Part model, mm, in its own coordinate system. Face numbers are marked on the shaded views. A direction names the side the tool comes from. Coordinates: 2 decimals unless noted, no trailing zeros. Use a Markdown table: item, result.
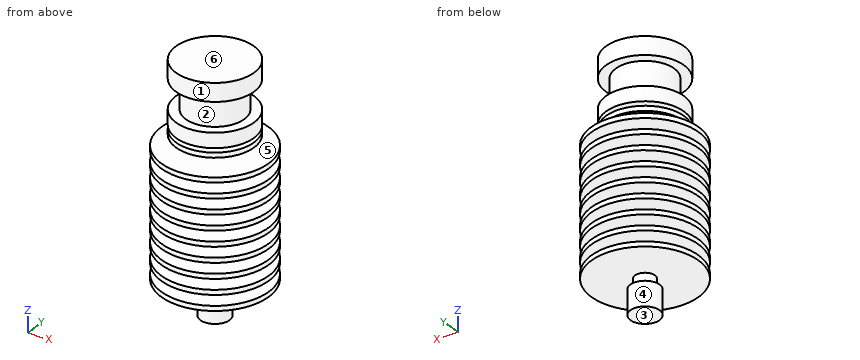
Autodesk Inventor part; units mm, degrees
ref_plane "YZ Plane" through (0, 0, 0) normal (1, 0, 0) x (0, 1, 0)
ref_plane "XZ Plane" through (0, 0, 0) normal (0, 1, 0) x (-1, 0, 0)
ref_plane "XY Plane" through (0, 0, 0) normal (0, 0, 1) x (1, 0, 0)
sketch "Sketch1" plane through (0, 0, 0) normal (1, 0, 0) x (0, 1, 0)
  line L0 (0, -49.8) -> (0, 0)
  line L1 (0, 0) -> (-8, 0)
  line L2 (-8, 0) -> (-8, -3.7)
  line L3 (-8, -3.7) -> (-6, -3.7)
  line L4 (-6, -3.7) -> (-6, -9.7)
  line L5 (-6, -9.7) -> (-8, -9.7)
  line L6 (-8, -9.7) -> (-8, -12.7)
  line L7 (-8, -12.7) -> (-3, -12.7)
  line L8 (-3, -12.7) -> (-3, -49.8)
  line L9 (-3, -49.8) -> (0, -49.8)
  line L10 (-3, -42.7) -> (-11, -42.7)
  line L11 (-11, -42.7) -> (-11, -41.7)
  line L12 (-11, -41.7) -> (-3, -41.7)
  line L13 (-3, -41.7) -> (-3, -42.7)
  line L14 (-3, -39.575) -> (-11, -39.575)
  line L15 (-11, -39.575) -> (-11, -38.575)
  line L16 (-11, -38.575) -> (-3, -38.575)
  line L17 (-3, -38.575) -> (-3, -39.575)
  line L18 (-3, -27.075) -> (-11, -27.075)
  line L19 (-11, -27.075) -> (-11, -26.075)
  line L20 (-11, -26.075) -> (-3, -26.075)
  line L21 (-3, -26.075) -> (-3, -27.075)
  line L22 (-3, -20.825) -> (-11, -20.825)
  line L23 (-11, -20.825) -> (-11, -19.825)
  line L24 (-11, -19.825) -> (-3, -19.825)
  line L25 (-3, -19.825) -> (-3, -20.825)
  line L26 (-3, -30.2) -> (-11, -30.2)
  line L27 (-11, -30.2) -> (-11, -29.2)
  line L28 (-11, -29.2) -> (-3, -29.2)
  line L29 (-3, -29.2) -> (-3, -30.2)
  line L30 (-3, -33.325) -> (-11, -33.325)
  line L31 (-11, -33.325) -> (-11, -32.325)
  line L32 (-11, -32.325) -> (-3, -32.325)
  line L33 (-3, -32.325) -> (-3, -33.325)
  line L34 (-3, -36.45) -> (-11, -36.45)
  line L35 (-11, -36.45) -> (-11, -35.45)
  line L36 (-11, -35.45) -> (-3, -35.45)
  line L37 (-3, -35.45) -> (-3, -36.45)
  line L38 (-3, -23.95) -> (-11, -23.95)
  line L39 (-11, -23.95) -> (-11, -22.95)
  line L40 (-11, -22.95) -> (-3, -22.95)
  line L41 (-3, -22.95) -> (-3, -23.95)
  line L42 (-3, -17.7) -> (-11, -17.7)
  line L43 (-11, -17.7) -> (-11, -16.7)
  line L44 (-11, -16.7) -> (-3, -16.7)
  line L45 (-3, -16.7) -> (-3, -17.7)
  line L46 (-11, -17.7) -> (-11, -19.825) construction
  line L47 (-11, -20.825) -> (-11, -22.95) construction
  line L48 (-11, -23.95) -> (-11, -26.075) construction
  line L49 (-11, -27.075) -> (-11, -29.2) construction
  line L50 (-11, -30.2) -> (-11, -32.325) construction
  line L51 (-11, -33.325) -> (-11, -35.45) construction
  line L52 (-11, -36.45) -> (-11, -38.575) construction
  line L53 (-11, -41.7) -> (-11, -39.575) construction
  line L54 (-8, -13.575) -> (-3, -13.575)
  line L55 (-3, -13.575) -> (-3, -14.575)
  line L56 (-3, -14.575) -> (-8, -14.575)
  line L57 (-8, -14.575) -> (-8, -13.575)
  line L58 (-8, -14.575) -> (-8, -16.7) construction
  line L59 (-3, -42.7) -> (-2.05, -42.7)
  line L60 (-2.05, -42.7) -> (-2.05, -44.8)
  line L61 (-2.05, -44.8) -> (-3, -44.8)
  line L62 (-3, -44.8) -> (-3, -42.7)
  dimension "d0" = 3.7
  dimension "d2" = 6
  dimension "d3" = 3
  dimension "d4" = 8
  dimension "d5" = 6
  dimension "d6" = 3
  dimension "d7" = 49.8
  dimension "d9" = 1
  dimension "d11" = 26
  dimension "d12" = 7.1
  dimension "d13" = 11
  dimension "d14" = 5
  dimension "d15" = 2.05
revolve "Revolution1" add sketch "Sketch1" angle 360 about axis through (0, 0, -49.8) along (0, 0, 1) contours L9 L8 L61 L60 L59 L7 L6 L5 L4 L3 L2 L1 L0 | L10 L11 L12 L8 | L14 L15 L16 L8 | L34 L35 L36 L8 | L8 L56 L57 L54 | L30 L31 L32 L8 | L8 L42 L43 L44 | L26 L27 L28 L8 | L8 L22 L23 L24 | L18 L19 L20 L8 | L8 L38 L39 L40
properties part number "heat sink"
Item 1: Band-saw the part on A-A, the plane y = -6.75. Count the separate pieces of the cut face and the enclosed holes in it, then the cut area to 3 significant figures.
From the geometry:
| item | result |
|---|---|
| separate pieces | 12 |
| enclosed holes | 0 |
| area | 222 mm^2 |
Item 2: Two-plate mould, pull along Z, no slides. Class the marked faces 4, 5 and 6: pulls with the +Z half, pulls with the -Z half, needs draft (parallel to the pull), parting line crosses it, or undercut.
From the geometry:
| item | result |
|---|---|
| face 4 | needs draft |
| face 5 | undercut |
| face 6 | pulls with the +Z half |
Item 3: Which spindle directions (+Z, -Z, +X, -X, +Y, -Y) get a long thin tool onto all of the face, cutting with end or side? Do the marked faces 1, 2 and 3. Say none if no direction does.
From the geometry:
| item | result |
|---|---|
| face 1 | +Z |
| face 2 | none |
| face 3 | -Z, +X, -X, +Y, -Y |
Item 4: Drop flat-ended pins along their axis: P1, Ø4, axis at y = -6.5, z = -10, coming from the +X side; P2, Ø10, axis at y = 4.5, z = -5, coming from the -X side; P3, Ø2, axis at y = 6, z = -31, coming from the -X side; P4, Ø1, axis at x = 8, z = -25, coming from the +Y side. Give the stop position or say it passes through.
From the geometry:
| item | result |
|---|---|
| P1 | x = 6.61 |
| P2 | x = -8 |
| P3 | x = -9.58 |
| P4 | through |
Item 5: Drill centre lines: probe 1 along Y at (x, z) = (0.25, -32); probe 2 along X at (y, z) = (0, -14); probe 3 along X at (y, z) = (10, -17). Where is each one in solid material? Low to high.
From the geometry:
| item | result |
|---|---|
| probe 1 | -2.99 to 2.99 |
| probe 2 | -8 to 8 |
| probe 3 | -4.58 to 4.58 |
